Read the model definition and answer for the solid it produces. Units are mm, in the model's axes. Coordinates: 2 decimals unless noted, no trailing zeros. Loops run counter-clockwise (first coordinate to the right, second up) from the corner with the lowest first, then second, coordinate; pieces in that order, holes last. Notation, with made-up numbers: M -2,73 L 42,73 A23 cw 42,103 Z; hole C 28,-17.75 d3. An arc over 180 degrees is marked long. Put each result on its own line as item: value.
from build123d import *

# Parameters (mm, degrees)
SKETCH1_R           = 1.5875
BOSS_EXTRUDE1_DEPTH = 1.5875
SKETCH2_R           = 3.175
SKETCH2_R_2         = 1.5875
BOSS_EXTRUDE2_DEPTH = 1.5875


with BuildPart() as part:
    # Sketch1 → Boss-Extrude1 (new body)
    with BuildSketch(Plane.XY):
        with BuildLine():
            Line((-34.953036507, -6.90745394), (-23.905143538, -44.62262411))
            ThreePointArc((-23.905143538, -44.62262411), (-26.059560971, -48.562133663), (-29.999070525, -46.407716231))
            Line((-29.999070525, -46.407716231), (-41.046963493, -8.69254606))
            ThreePointArc((-41.046963493, -8.69254606), (-38.89254606, -4.753036507), (-34.953036507, -6.90745394))
        make_face()
        with Locations((-26.952107032, -45.51517017)):
            Circle(SKETCH1_R, mode=Mode.SUBTRACT)
        with Locations((-38, -7.8)):
            Circle(SKETCH1_R, mode=Mode.SUBTRACT)
    extrude(amount=BOSS_EXTRUDE1_DEPTH)

    # Sketch2 → Boss-Extrude2 (add)
    with BuildSketch(Plane.XY.offset(1.5875)):
        with Locations(Location((-38, -7.8, 0), (0, 0, 196.32687427))):
            Circle(SKETCH2_R)
        with Locations((-38, -7.8)):
            Circle(SKETCH2_R_2, mode=Mode.SUBTRACT)
    extrude(amount=BOSS_EXTRUDE2_DEPTH)


solid = part.part
1) Straight lines are drawn through the part: line 1 (Y direction, x = -38, z = 1.85) (1 decimal); line 2 (Y direction, x = -37.25, z = 1.75); line 3 (X direction, y = -20, z = 1.15). For each, find the intervals that lie inside material, in ascending order. Write a range as [from, to].
Answer list:
line 1: y = [-11, -9.4], [-6.2, -4.6]
line 2: y = [-10.89, -9.2], [-6.4, -4.71]
line 3: x = [-37.73, -31.12]
2) Find section B-B, the plane x = -38. Write down the section's boundary in (y, z) (1 decimal), plus the area to 3 significant figures.
Answer list:
outline: M -19.1,0 L -9.4,0 L -9.4,3.2 L -11,3.2 L -11,1.6 L -19.1,1.6 Z; M -6.2,0 L -4.6,0 L -4.6,3.2 L -6.2,3.2 Z
area: 23.0 mm^2
3) Given pin 1 Ø5 at (x, y) = (-26.95, -45.52) entering from +Z, flat-ended and moving along its own axis, determine where the tip first touches the part or whether it passes through.
Answer list:
pin 1: stops at z = 1.59
4) Determine the mould class of faces 1 (the cylindrical face through (-27.296, -47.065, 0.783)), 2 (the flat face through (-35.446, -27.814, 0.783)), 3 (the flat face through (-32, -28, 0)) for opening direction X: released by +X, released by -X, zero draft, split by the parting line, or undercut.
Answer list:
face 1: undercut
face 2: released by -X
face 3: zero draft
5) Find section D-D, the plane z = 0.6. Count the separate pieces of the cut face and the enclosed holes in it, plus the area to 3 significant figures.
Answer list:
separate pieces: 1
enclosed holes: 2
area: 265 mm^2
